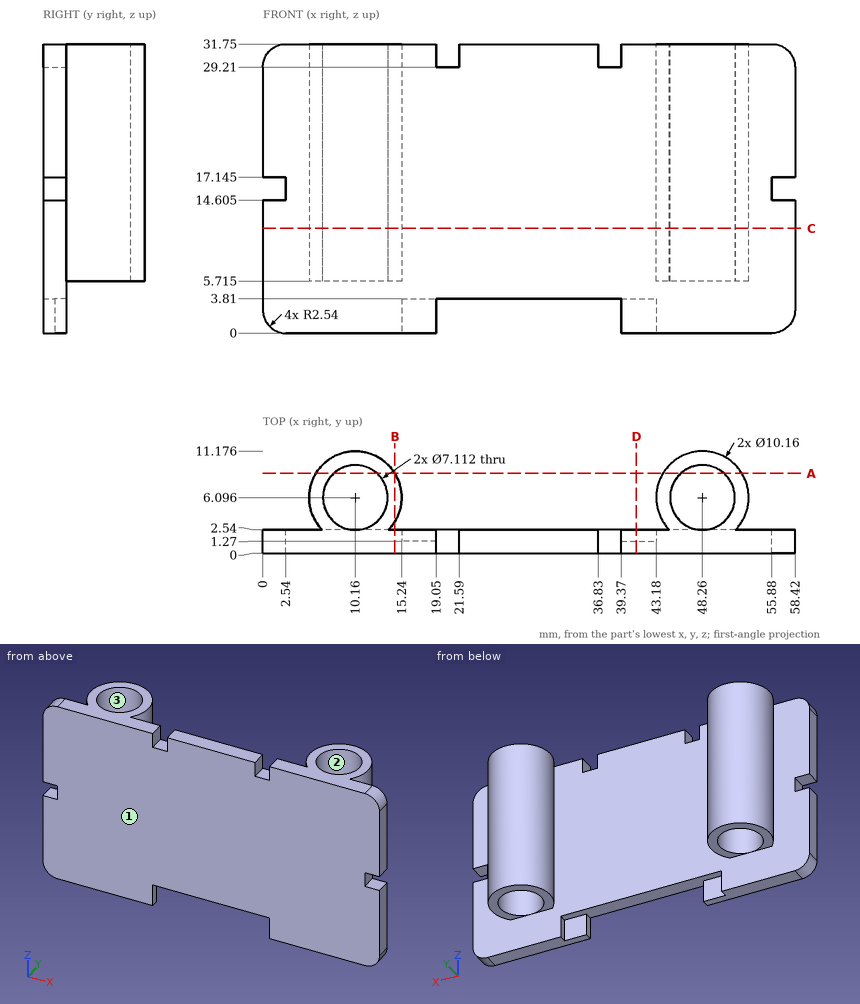
Job drawing, mm, ordinate dimensions from the low corner. One solid piece. Coordinates: 2 decimals unless noted, no trailing zeros. Order: outer loops, then holes, each group sorted by start corner. A loop starts at its lowest first (then second) coordinate and runs counter-clockwise, first axis right, second up. Notation, with made-up numbers: (-5, 51.25) - (29, 51.25) arc R19 ccw to (29, 63.25) - close; hole circle Ø5 at (83, 24.5). An arc over 180 degrees is marked (long way). Write each question's results on one line, items separated by ' | '. Start each with the question number.
Item 1: Wall check: probe 1 along Y at (x, z) = (10, 15.5); probe 2 along X at (y, z) = (8.5, 7); probe 3 along X at (y, z) = (3.25, 29). Give the ranges that are in metal, low to high. Write a range as [from, to].
Item 2: Mould opens along X. For the marked faces 1, 2 and 3 say: released by +X, released by -X, zero draft, split by the parting line, or undercut.
Item 3: Band-saw the part on C-C on z = 11.5. Write the cut outline in (x, y), and give its area (3 significant figures).
Item 4: Band-saw the part on A-A on y = 8.75. Write the cut outline in (x, z) (3 decimals), and give its area (3 significant figures).
Item 5: Band-saw the part on B-B on x = 14.5. Write the cut outline in (y, z) (3 decimals), and give its area (3 significant figures).
Item 6: Band-saw the part on D-D on x = 41. Write the cut outline in (y, z), and give its area (3 significant figures).
Item 7: Flat gauge pins, fed straight in: pin 1 (0.6 mm diameter, centred on y = 0.5, z = 1.5, fed in from +X); pin 2 (2 mm diameter, centred on y = 4.5, z = 3.5, fed in from -X); pin 3 (0.8 mm diameter, centred on x = 38, y = 0.5, fed in from +Z); pin 4 (0.8 mm diameter, centred on x = 57.5, y = 1.5, fed in from -Z). Where does each tip first touch, or does it go through?
Numbers:
1) probe 1: [0, 2.54], [9.65, 11.17] | probe 2: [5.68, 7.54], [12.78, 14.64], [43.78, 45.64], [50.88, 52.74] | probe 3: [5.95, 8.03], [12.29, 14.37], [44.05, 46.13], [50.39, 52.47]
2) face 1: zero draft | face 2: undercut | face 3: undercut
3) outline: (0, 0) - (58.42, 0) - (58.42, 2.54) - (51.89, 2.54) arc R5.08 ccw (long way) to (44.63, 2.54) - (13.79, 2.54) arc R5.08 ccw (long way) to (6.53, 2.54) - (0, 2.54) - close; hole circle Ø7.11 at (10.16, 6.1); hole circle Ø7.11 at (48.26, 6.1) | area: 216 mm^2
4) outline: (5.828, 5.715) - (7.793, 5.715) - (7.793, 31.75) - (5.828, 31.75) - close; (12.527, 5.715) - (14.492, 5.715) - (14.492, 31.75) - (12.527, 31.75) - close; (43.928, 5.715) - (45.893, 5.715) - (45.893, 31.75) - (43.928, 31.75) - close; (50.627, 5.715) - (52.592, 5.715) - (52.592, 31.75) - (50.627, 31.75) - close | area: 205 mm^2
5) outline: (0, 0) - (2.54, 0) - (2.54, 31.75) - (0, 31.75) - close; (3.456, 5.715) - (8.736, 5.715) - (8.736, 31.75) - (3.456, 31.75) - close | area: 218 mm^2
6) outline: (0, 0) - (1.27, 0) - (1.27, 3.81) - (2.54, 3.81) - (2.54, 31.75) - (0, 31.75) - close | area: 75.8 mm^2
7) pin 1: x = 58.31 | pin 2: through | pin 3: z = 29.21 | pin 4: z = 0.31
